from build123d import *

# Parameters (mm, degrees)
SKETCH1_R           = 5
BOSS_EXTRUDE1_DEPTH = 1.4
BOSS_EXTRUDE2_DEPTH = 0.8


with BuildPart() as part:
    # Sketch1 → Boss-Extrude1 (new body)
    with BuildSketch(Plane.XY):
        with BuildLine():
            Line((20, 60), (20, 62.81))
            ThreePointArc((20, 62.81), (18.828427125, 65.638427125), (16, 66.81))
            Line((16, 66.81), (-16, 66.81))
            ThreePointArc((-16, 66.81), (-18.828427125, 65.638427125), (-20, 62.81))
            Line((-20, 62.81), (-20, 60))
            ThreePointArc((-20, 60), (-21.464466094, 56.464466094), (-25, 55))
            Line((-25, 55), (-27.81, 55))
            ThreePointArc((-27.81, 55), (-30.638427125, 53.828427125), (-31.81, 51))
            Line((-31.81, 51), (-31.81, -51))
            ThreePointArc((-31.81, -51), (-30.638427125, -53.828427125), (-27.81, -55))
            Line((-27.81, -55), (-25, -55))
            ThreePointArc((-25, -55), (-21.464466094, -56.464466094), (-20, -60))
            Line((-20, -60), (-20, -62.81))
            ThreePointArc((-20, -62.81), (-18.828427125, -65.638427125), (-16, -66.81))
            Line((-16, -66.81), (16, -66.81))
            ThreePointArc((16, -66.81), (18.828427125, -65.638427125), (20, -62.81))
            Line((20, -62.81), (20, -60))
            ThreePointArc((20, -60), (21.464466094, -56.464466094), (25, -55))
            Line((25, -55), (27.81, -55))
            ThreePointArc((27.81, -55), (30.638427125, -53.828427125), (31.81, -51))
            Line((31.81, -51), (31.81, 51))
            ThreePointArc((31.81, 51), (30.638427125, 53.828427125), (27.81, 55))
            Line((27.81, 55), (25, 55))
            ThreePointArc((25, 55), (21.464466094, 56.464466094), (20, 60))
        make_face()
        with Locations((-25, 10)):
            Circle(SKETCH1_R, mode=Mode.SUBTRACT)
        with Locations((25, 10)):
            Circle(SKETCH1_R, mode=Mode.SUBTRACT)
        with Locations((-25, -10)):
            Circle(SKETCH1_R, mode=Mode.SUBTRACT)
        with Locations((25, -10)):
            Circle(SKETCH1_R, mode=Mode.SUBTRACT)
    extrude(amount=BOSS_EXTRUDE1_DEPTH)

    # Sketch2 → Boss-Extrude2 (add)
    with BuildSketch(Plane.XY.offset(1.4)):
        with BuildLine():
            Line((-24.048951294, 37.5), (-14.735982135, 37.5))
            ThreePointArc((-14.735982135, 37.5), (-13.281012897, 37.967006022), (-12.369627175, 39.193548387))
            ThreePointArc((-12.369627175, 39.193548387), (-9.256969539, 44.192388155), (-4.258129771, 47.305045791))
            ThreePointArc((-4.258129771, 47.305045791), (-3.031587405, 48.216431513), (-2.564581384, 49.671400751))
            Line((-2.564581384, 49.671400751), (-2.564581384, 58.98436991))
            ThreePointArc((-2.564581384, 58.98436991), (-3.487481229, 60.924152141), (-5.574785465, 61.431754595))
            ThreePointArc((-5.574785465, 61.431754595), (-19.156464476, 54.091883092), (-26.496335979, 40.510204082))
            ThreePointArc((-26.496335979, 40.510204082), (-25.988733525, 38.422899845), (-24.048951294, 37.5))
        make_face()
        with BuildLine():
            Line((23.919788527, 37.5), (14.606819368, 37.5))
            ThreePointArc((14.606819368, 37.5), (13.151850129, 37.967006022), (12.240464408, 39.193548387))
            ThreePointArc((12.240464408, 39.193548387), (9.127806772, 44.192388155), (4.128967004, 47.305045791))
            ThreePointArc((4.128967004, 47.305045791), (2.902424638, 48.216431513), (2.435418616, 49.671400751))
            Line((2.435418616, 49.671400751), (2.435418616, 58.98436991))
            ThreePointArc((2.435418616, 58.98436991), (3.358318462, 60.924152141), (5.445622698, 61.431754595))
            ThreePointArc((5.445622698, 61.431754595), (19.027301709, 54.091883092), (26.367173212, 40.510204082))
            ThreePointArc((26.367173212, 40.510204082), (25.859570757, 38.422899845), (23.919788527, 37.5))
        make_face()
        with BuildLine():
            Line((-24.048951294, -37.5), (-14.735982135, -37.5))
            ThreePointArc((-14.735982135, -37.5), (-13.281012897, -37.967006022), (-12.369627175, -39.193548387))
            ThreePointArc((-12.369627175, -39.193548387), (-9.256969539, -44.192388155), (-4.258129771, -47.305045791))
            ThreePointArc((-4.258129771, -47.305045791), (-3.031587405, -48.216431513), (-2.564581384, -49.671400751))
            Line((-2.564581384, -49.671400751), (-2.564581384, -58.98436991))
            ThreePointArc((-2.564581384, -58.98436991), (-3.487481229, -60.924152141), (-5.574785465, -61.431754595))
            ThreePointArc((-5.574785465, -61.431754595), (-19.156464476, -54.091883092), (-26.496335979, -40.510204082))
            ThreePointArc((-26.496335979, -40.510204082), (-25.988733525, -38.422899845), (-24.048951294, -37.5))
        make_face()
        with BuildLine():
            Line((2.435418616, -49.671400751), (2.435418616, -58.98436991))
            ThreePointArc((2.435418616, -58.98436991), (3.358318462, -60.924152141), (5.445622698, -61.431754595))
            ThreePointArc((5.445622698, -61.431754595), (19.027301709, -54.091883092), (26.367173212, -40.510204082))
            ThreePointArc((26.367173212, -40.510204082), (25.859570757, -38.422899845), (23.919788527, -37.5))
            Line((23.919788527, -37.5), (14.606819368, -37.5))
            ThreePointArc((14.606819368, -37.5), (13.151850129, -37.967006022), (12.240464408, -39.193548387))
            ThreePointArc((12.240464408, -39.193548387), (9.127806772, -44.192388155), (4.128967004, -47.305045791))
            ThreePointArc((4.128967004, -47.305045791), (2.902424638, -48.216431513), (2.435418616, -49.671400751))
        make_face()
    extrude(amount=BOSS_EXTRUDE2_DEPTH)


solid = part.part
CAD build for the part. Positions are in the model's coordinates, mm. A direction names the side the tool comes from. Give positions to 0.01 mm unless a question says otherwise; leave off trailing zeros. Write each loop counter-clockwise with the first axis right and the second up, starting at its lowest first coordinate (ties: lowest second). Pieces come first, ordered by that corner, then holes. Notation, with made-up numbers: M 46,-19 L 100,-19 A14 cw 100,-12 Z; hole C 71,8 d9. An arc over 180 degrees is marked long. Put each result on its own line as item: value. Start each with the question number.
(1) Mould opens along X. For faces 1 (the face through (-30.607, 53.859, 0.69)), 2 (the face through (22, 56, 1)), 3 (the face through (-30, 10, 1)), 4 (the face through (14, -49, 2.2)) say: +X half, -X half, draft (parallel to the pull), parting line (faces both ways), or undercut.
(2) Which spindle directions (+Z, -Z, +X, -X, +Y, -Y) get a long thin tool onto all of the face, cutting with end or side? Do faces 5 (the face through (18.87, -54.25, 1.79)), 6 (the face through (18.87, 54.25, 1.79)), 7 (the face through (-26.01, 38.45, 1.79)), 8 (the face through (25.88, -38.45, 1.79)), 9 (the face through (3.33, -60.9, 1.79)). Say none if no direction does.
(3) Flat gauge pins, fed straight in: pin 1 Ø1.1 at (x, z) = (-26, 1) entering from -Y; pin 2 Ø1.1 at (y, z) = (62, 1) entering from +X; pin 3 Ø4 at (x, y) = (-14, -2.5) entering from +Z. Where does each tip first touch, or does it go through?
(4) Probe L1, parallel to Y at x = -25, z = 0.8; L2, parallel to Y at x = -23, z = 0.65; L3, parallel to Z at x = 8.5, y = 43. List the from-to ranges inside material, lowest first.
(5) Band-saw the part on B-B, the plane z = 0.8. Write the cut outline in (x, y).
(6) Band-saw the part on D-D, the plane y = -44. Write the cut outline in (x, z).
(7) Band-saw the part on A-A, the plane y = -10. Write the cut outline in (x, z).
(8) Band-saw the part on C-C, the plane x = 8.5. Write the cut outline in (y, z).
Response values:
1. face 1: -X half
1. face 2: +X half
1. face 3: undercut
1. face 4: draft
2. face 5: +Z, +X, -Y
2. face 6: +Z, +X, +Y
2. face 7: +Z, -X
2. face 8: +Z, +X
2. face 9: +Z, -Y
3. pin 1: stops at y = -55
3. pin 2: stops at x = 20
3. pin 3: stops at z = 1.4
4. L1: y = -55 to -15, -5 to 5, 15 to 55
4. L2: y = -55.42 to -14.58, -5.42 to 5.42, 14.58 to 55.42
4. L3: z = 0 to 1.4
5. outline: M -31.81,-51 A4 ccw -27.81,-55 L -25,-55 A5 cw -20,-60 L -20,-62.81 A4 ccw -16,-66.81 L 16,-66.81 A4 ccw 20,-62.81 L 20,-60 A5 cw 25,-55 L 27.81,-55 A4 ccw 31.81,-51 L 31.81,51 A4 ccw 27.81,55 L 25,55 A5 cw 20,60 L 20,62.81 A4 ccw 16,66.81 L -16,66.81 A4 ccw -20,62.81 L -20,60 A5 cw -25,55 L -27.81,55 A4 ccw -31.81,51 Z; hole C -25,-10 d10; hole C -25,10 d10; hole C 25,-10 d10; hole C 25,10 d10
6. outline: M -31.81,0 L 31.81,0 L 31.81,1.4 L 25.39,1.4 L 25.39,2.2 L 9.32,2.2 L 9.32,1.4 L -9.45,1.4 L -9.45,2.2 L -25.52,2.2 L -25.52,1.4 L -31.81,1.4 Z
7. outline: M -31.81,0 L -30,0 L -30,1.4 L -31.81,1.4 Z; M -20,0 L 20,0 L 20,1.4 L -20,1.4 Z; M 30,0 L 31.81,0 L 31.81,1.4 L 30,1.4 Z
8. outline: M -66.81,0 L 66.81,0 L 66.81,1.4 L 60.61,1.4 L 60.61,2.2 L 44.78,2.2 L 44.78,1.4 L -44.78,1.4 L -44.78,2.2 L -60.61,2.2 L -60.61,1.4 L -66.81,1.4 Z
